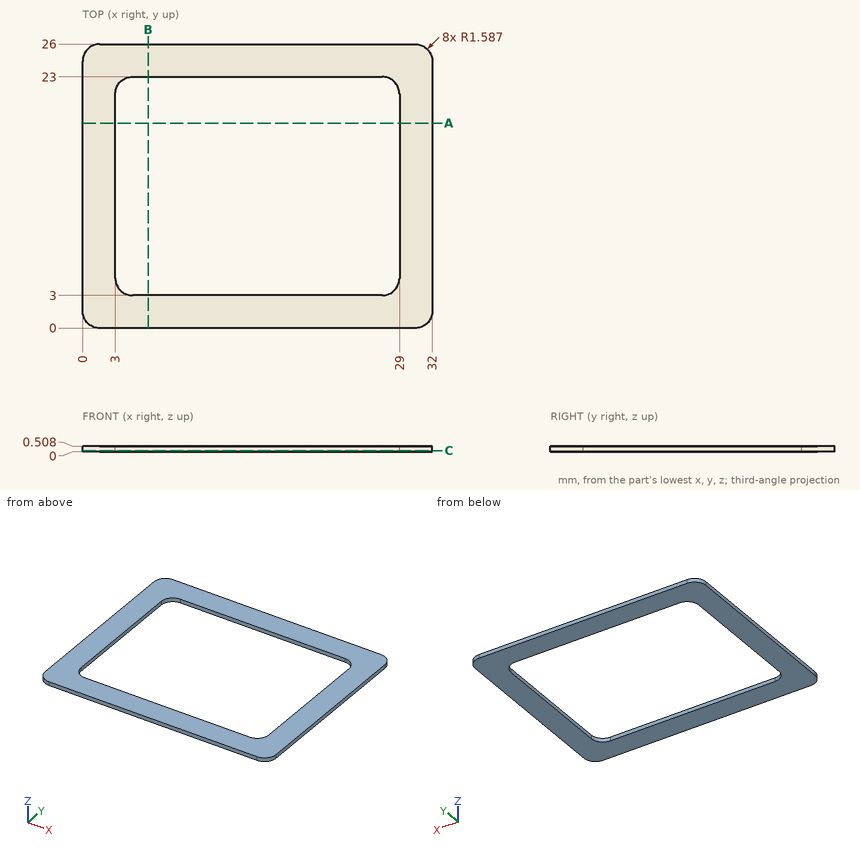
The drawing under review shows one solid part. Ordinate dimensions are in mm from its lowest x, y, z. Give positions to 0.01 mm unless a question says otherwise; leave off trailing zeros. Loops run counter-clockwise (first coordinate to the right, second up) from the corner with the lowest first, then second, coordinate; pieces in that order, holes last. Notation, with made-up numbers: M -17.75,13 L 19.25,13 A18 cw 19.25,38 Z; hole C -30,76 d5. An arc over 180 degrees is marked long. Return JSON: item names as keys, results as strings. Group by question number.
Item 1: For probe 1 along X at (y, z) = (9.75, 0.1); probe 2 along Y at (x, z) = (20, 0.3); probe 3 along X at (y, z) = (3.75, 0.15), list the stretches that pass through material, from the lowest coordinate up.
Item 2: We need section A-A (y = 18.75). Give the boundary of the cut face in (x, z).
Item 3: We need section C-C (z = 0.1). Give the boundary of the cut face in (x, y) (1 decimal), and give its area (3 significant figures).
Item 4: We need section B-B (x = 6). Give the boundary of the cut face in (y, z).
Output:
{
 "1": {"probe 1": "x = 0 to 3, 29 to 32", "probe 2": "y = 0 to 3, 23 to 26", "probe 3": "x = 0 to 3.24, 28.76 to 32"},
 "2": {"outline": "M 0,0 L 3,0 L 3,0.51 L 0,0.51 Z; M 29,0 L 32,0 L 32,0.51 L 29,0.51 Z"},
 "3": {"outline": "M 0,1.6 A1.6 ccw 1.6,0 L 30.4,0 A1.6 ccw 32,1.6 L 32,24.4 A1.6 ccw 30.4,26 L 1.6,26 A1.6 ccw 0,24.4 Z; hole M 3,4.6 A1.6 ccw 4.6,3 L 27.4,3 A1.6 ccw 29,4.6 L 29,21.4 A1.6 ccw 27.4,23 L 4.6,23 A1.6 ccw 3,21.4 Z", "area": "312 mm^2"},
 "4": {"outline": "M 0,0 L 3,0 L 3,0.51 L 0,0.51 Z; M 23,0 L 26,0 L 26,0.51 L 23,0.51 Z"}
}
